Input: part model. Units: mm. Frame: model coordinates. Face numbers are marked on the shaded views. Give positions to 0.01 mm unless a question says otherwise; leave off trailing zeros. Write each loop counter-clockwise with the first axis right and the second up, starting at its lowest first coordinate (ties: lowest second). Pieces come first, ordered by that corner, then holes. Notation, with made-up numbers: (-33, 2) - (-2, 2) arc R18 ccw to (-2, 23) - close; hole circle Ø2 at (-25.75, -4.75). An arc over 180 degrees is marked (long way). Use a Markdown table: item, result. Add a question column.
1. Section query D-D, the plane x = -9. Return loops of the section in (y, z), plus the area to 3 significant figures.
2. Material intervals for probe 1 along Z at (x, y) = (0, 4.25); probe 2 along X at (y, z) = (4.5, 0); probe 3 along Y at (x, z) = (2, -0.5), sorted ascending.
3. Mould query, pull axis X, two halves, no side actions, for the marked faces 1, 2, 3 and 4. Classes: released by +X, released by -X, zero draft, split by the parting line, or undercut.
4. Pin query (flat end, axial travel): pin 1 (6 mm diameter, centred on x = -1.5, z = -4.5, fed in from -Y); pin 2 (10 mm diameter, centred on y = 18.5, z = -2.5, fed in from +X); pin 3 (1 mm diameter, centred on x = -6, y = 25, fed in from -Z); pin 4 (5 mm diameter, centred on x = 5.5, y = 24, fed in from +Z). Return the tip coordinate at first contact, or that it passes through.
5. Section query C-C, the plane y = 15. Return loops of the section in (x, z), plus the area to 3 significant figures.
6. Section query A-A, the plane x = 0. Return loops of the section in (y, z).
7. Section query B-B, the plane z = -9.5. Return loops of the section in (x, y), plus the area to 3 significant figures.
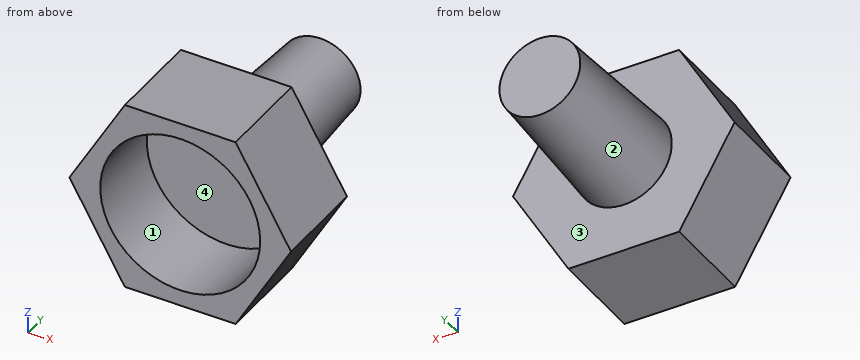
```python
from build123d import *

# Parameters (mm, degrees)
BOSS_EXTRUDE1_DEPTH = 12
BOSS_EXTRUDE2_START = 12
SKETCH2_R           = 6
BOSS_EXTRUDE2_DEPTH = 18
BOSS_EXTRUDE2_TAPER = 3
SKETCH3_R           = 10
CUT_EXTRUDE1_DEPTH  = 10


with BuildPart() as part:
    # Sketch1 → Boss-Extrude1 (new body)
    with BuildSketch(Plane(origin=(0, 0, 0), x_dir=(1, 0, 0), z_dir=(0, 1, 0))):
        Polygon((13.856406461, 0), (6.92820323, 12), (-6.92820323, 12), (-13.856406461, 0), (-6.92820323, -12), (6.92820323, -12), align=None)
    extrude(amount=BOSS_EXTRUDE1_DEPTH)

    # Sketch2 → Boss-Extrude2 (add)
    with BuildSketch(Plane(origin=(0, 0, 0), x_dir=(1, 0, 0), z_dir=(0, 1, 0)).offset(BOSS_EXTRUDE2_START)):
        Circle(SKETCH2_R)
    extrude(amount=BOSS_EXTRUDE2_DEPTH, taper=BOSS_EXTRUDE2_TAPER)

    # Sketch3 → Cut-Extrude1 (cut)
    with BuildSketch(Plane(origin=(0, 0, 0), x_dir=(1, 0, 0), z_dir=(0, 1, 0))):
        Circle(SKETCH3_R)
    extrude(amount=CUT_EXTRUDE1_DEPTH, mode=Mode.SUBTRACT)


solid = part.part
```
Result sheet:
| question | item | result |
|---|---|---|
| 1 | outline | (0, -8.41) - (12, -8.41) - (12, 8.41) - (0, 8.41) - (0, 4.36) - (10, 4.36) - (10, -4.36) - (0, -4.36) - close |
| 1 | area | 115 mm² |
| 2 | probe 1 | z = -12 to -10, 10 to 12 |
| 2 | probe 2 | x = -13.86 to -10, 10 to 13.86 |
| 2 | probe 3 | y = 10 to 30 |
| 3 | face 1 | undercut |
| 3 | face 2 | split by the parting line |
| 3 | face 3 | zero draft |
| 3 | face 4 | undercut |
| 4 | pin 1 | stops at y = 10 |
| 4 | pin 2 | stops at x = 5.89 |
| 4 | pin 3 | passes through |
| 4 | pin 4 | stops at z = 4.46 |
| 5 | outline | circle Ø11.69 at (0, 0) |
| 5 | area | 107 mm² |
| 6 | outline | (0, -12) - (12, -12) - (12, -6) - (30, -5.06) - (30, 5.06) - (12, 6) - (12, 12) - (0, 12) - (0, 10) - (10, 10) - (10, -10) - (0, -10) - close |
| 7 | outline | (-8.37, 0) - (-3.12, 0) - (-3.12, 10) - (3.12, 10) - (3.12, 0) - (8.37, 0) - (8.37, 12) - (-8.37, 12) - close |
| 7 | area | 138 mm² |
